Geometry check sheet. Reference: drawing and pictorial views, mm from the part's lowest x, y, z. A direction names the side the tool comes from. Coordinates: 2 decimals unless noted, no trailing zeros. Write each loop counter-clockwise with the first axis right and the second up, starting at its lowest first coordinate (ties: lowest second). Pieces come first, ordered by that corner, then holes. Notation, with made-up numbers: (-23, 52) - (29, 52) arc R7 cw to (29, 56) - close; hole circle Ø10 at (19.5, 18). An arc over 180 degrees is marked (long way). Use one line per item in the form item = value. Start each with the question number.
(1) Sectioned sample at C-C (y = 4.7). Record the cut outline in (x, z).
(2) Sectioned sample at B-B (z = 9). Record the cut outline in (x, y).
(3) Gauge pin test, flat ends, axial feed: pin 1 Ø5 at (y, z) = (19.5, 5) entering from -X; pin 2 Ø1 at (y, z) = (12, 13.5) entering from -X (1 decimal); pin 3 Ø5 at (x, y) = (14, 5.5) entering from -Z (1 decimal). Record the tip position at first contact, or that the pin passes through.
(4) Sectioned sample at D-D (y = 35). Record the cut outline in (x, z).
(5) Material ranges on line 1 (X direction, y = 15, z = 9); line 2 (Y direction, x = 16.25, z = 8.5); line 3 (Z direction, x = 6.25, y = 13.5), recorded low to high. Write a range as [from, to].
(6) Sectioned sample at A-A (x = 9). Record the cut outline in (y, z).
(7) Mould release check, pull along Z, two halves, no side actions. Record for the marked faces 3, 4 and 5: released by +Z, released by -Z, zero draft, split by the parting line, or undercut.
(8) Tool access check on the marked faces 1 and 2. Record the directions out of +Z, -Z, +X, -X, +Y, -Y that give a thin tool (end or side, any length) a straight path to the whole face; none if there is none.
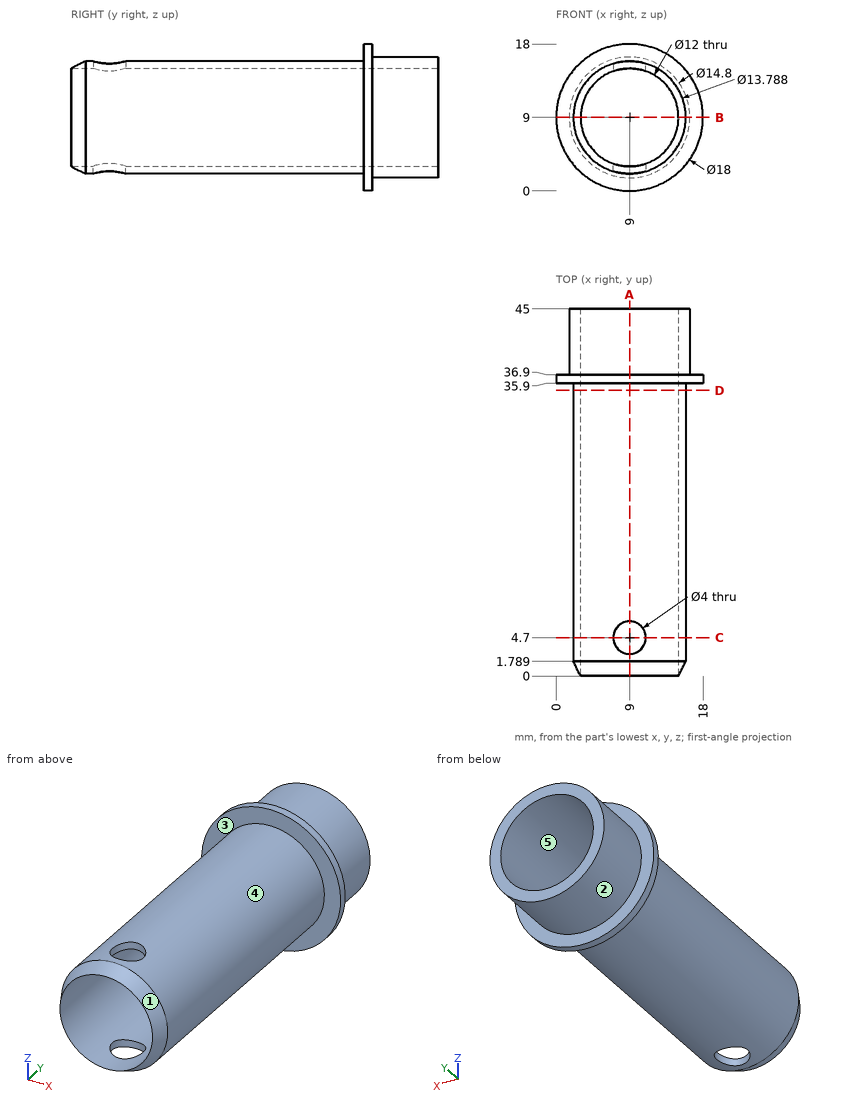
Answers below:
q1.outline = (7, 2.4) - (7, 3.34) arc R6 cw to (7, 14.66) - (7, 15.6) arc R6.89 ccw to start; (11, 2.4) arc R6.89 ccw to (11, 15.6) - (11, 14.66) arc R6 cw to (11, 3.34) - close
q2.outline = (0, 35.9) - (2.11, 35.9) - (2.11, 1.79) - (3, 0) - (3, 45) - (1.6, 45) - (1.6, 36.9) - (0, 36.9) - close; (15, 0) - (15.89, 1.79) - (15.89, 35.9) - (18, 35.9) - (18, 36.9) - (16.4, 36.9) - (16.4, 45) - (15, 45) - close
q3.pin_1 = 2.27
q3.pin_2 = 3.4
q3.pin_3 = 2.6
q4.outline = circle Ø13.79 at (9, 9); hole circle Ø12 at (9, 9)
q5.line_1 = [2.11, 3], [15, 15.89]
q5.line_2 = [35.9, 45]
q5.line_3 = [2.68, 3.67], [14.33, 15.32]
q6.outline = (0, 3) - (1.79, 2.11) - (2.7, 2.11) - (2.7, 3) - close; (0, 15) - (2.7, 15) - (2.7, 15.89) - (1.79, 15.89) - close; (6.7, 2.11) - (35.9, 2.11) - (35.9, 0) - (36.9, 0) - (36.9, 1.6) - (45, 1.6) - (45, 3) - (6.7, 3) - close; (6.7, 15) - (45, 15) - (45, 16.4) - (36.9, 16.4) - (36.9, 18) - (35.9, 18) - (35.9, 15.89) - (6.7, 15.89) - close
q7.face_3 = zero draft
q7.face_4 = split by the parting line
q7.face_5 = undercut
q8.face_1 = -Y
q8.face_2 = +Y
